Work out the finished part from the listing and answer in its coordinate system (mm). Face numbers are marked on the shaded views. A direction names the side the tool comes from. Coordinates: 2 decimals unless noted, no trailing zeros. Order: outer loops, then holes, each group sorted by start corner. A loop starts at its lowest first (then second) coordinate and runs counter-clockwise, first axis right, second up. Notation, with made-up numbers: (-19.5, -26) - (0.5, -26) arc R25 ccw to (0.5, -8) - close; hole circle Ø10 at (42.5, 48). An arc over 180 degrees is marked (long way). Answer as a JSON object with one key per item and string values. Group by question number.
1) A tool of negligible diameter and unlimited length cuts with its end or side. For the marked faces 1 and 2, from which of +Z, -Z, +X, -X, +Y, -Y can it reach the whole face along a straight path? Write none if from no direction.
2) Section D-D (x = -19.5) is taken. Give the vertices of the cut face in (y, z).
3) Section A-A (x = 0) is taken. Give the vertices of the cut face in (y, z).
4) Each of these flat-tipped pins is pushed along its axis until it touches: P1, Ø1.5, axis at y = 5, z = 11, coming from the -X side; P2, Ø8, axis at x = -12, y = 0, coming from the -Z side; P3, Ø4, axis at y = -12.5, z = 12.5, coming from the -X side. Where does it stop, or does it pass through?
5) Section C-C (y = -13) is taken. Give the vertices of the cut face in (x, z).
6) Section B-B (z = 0) is taken. Give the vertices of the cut face in (x, y).
7) Find the intervals of material crossed by line 1 along Y through (x, z) = (17, -8.5); line 2 along X through (y, z) = (-6.5, 0); line 3 along Z through (x, y) = (-12.5, 4.5), in increasing order.
8) The mould has two halves that part along X. Classify the marked faces 3, 4 and 5: released by +X, released by -X, zero draft, split by the parting line, or undercut.
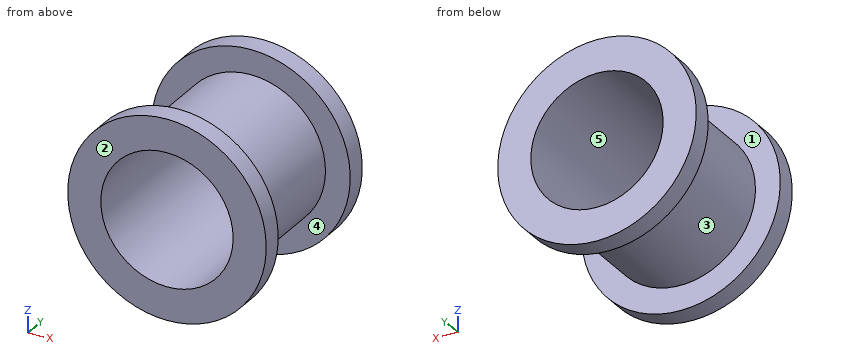
from build123d import *

# Parameters (mm, degrees)
SKETCH1_R           = 18
EXTRUDE1_DEPTH      = 15
SKETCH2_R           = 24
EXTRUDE2_DEPTH      = 5
EXTRUDE4_DEPTH      = 40.395431207
EXTRUDE4_DEPTH_BACK = 40.395431207
SKETCH3_R           = 16


with BuildPart() as part:
    # Sketch1 → Extrude1 (new, symmetric)
    with BuildSketch(Plane(origin=(0, 0, 0), x_dir=(1, 0, 0), z_dir=(0, 1, 0))):
        with Locations(Location((0, 0, 0), (0, 0, 270))):
            Circle(SKETCH1_R)
    extrude(amount=EXTRUDE1_DEPTH, both=True)

    # Sketch2 → Extrude2 (add)
    with BuildSketch(Plane(origin=(0, 15, 0), x_dir=(1, 0, 0), z_dir=(0, 1, 0))):
        with Locations(Location((0, 0, 0), (0, 0, 270))):
            Circle(SKETCH2_R)
    extrude2 = extrude(amount=EXTRUDE2_DEPTH)

    # Mirror1: Extrude2 across plane
    add(extrude2.mirror(Plane.ZX))

    # Sketch3 → Extrude4 (cut, two sides: drawn at the far end of the back side and taken through both)
    with BuildSketch(Plane(origin=(0, 0, 0), x_dir=(1, 0, 0), z_dir=(0, 1, 0)).offset(-EXTRUDE4_DEPTH_BACK)):
        with Locations(Location((0, 0, 0), (0, 0, 270))):
            Circle(SKETCH3_R)
    extrude(amount=EXTRUDE4_DEPTH + EXTRUDE4_DEPTH_BACK, mode=Mode.SUBTRACT)


solid = part.part
Report:
{
 "1": {"face 1": "none", "face 2": "+Z, -Z, +X, -X, -Y"},
 "2": {"outline": "(-20, -13.99) - (-15, -13.99) - (-15, 13.99) - (-20, 13.99) - close; (15, -13.99) - (20, -13.99) - (20, 13.99) - (15, 13.99) - close"},
 "3": {"outline": "(-20, -24) - (-15, -24) - (-15, -18) - (15, -18) - (15, -24) - (20, -24) - (20, -16) - (-20, -16) - close; (-20, 16) - (20, 16) - (20, 24) - (15, 24) - (15, 18) - (-15, 18) - (-15, 24) - (-20, 24) - close"},
 "4": {"P1": "stops at x = -14.8", "P2": "stops at z = -16.12", "P3": "stops at x = -14.62"},
 "5": {"outline": "circle Ø36 at (0, 0); hole circle Ø32 at (0, 0)"},
 "6": {"outline": "(-24, -20) - (-16, -20) - (-16, 20) - (-24, 20) - (-24, 15) - (-18, 15) - (-18, -15) - (-24, -15) - close; (16, -20) - (24, -20) - (24, -15) - (18, -15) - (18, 15) - (24, 15) - (24, 20) - (16, 20) - close"},
 "7": {"line 1": "y = -20 to -15, 15 to 20", "line 2": "x = -18 to -16, 16 to 18", "line 3": "z = -12.95 to -9.99, 9.99 to 12.95"},
 "8": {"face 3": "split by the parting line", "face 4": "zero draft", "face 5": "undercut"}
}
